```python
from build123d import *

# Parameters (mm, degrees)
SKETCH1_R           = 19.05
BOSS_EXTRUDE1_DEPTH = 34.29
SKETCH3_R           = 10.16
BOSS_EXTRUDE3_DEPTH = 5.08
BOSS_EXTRUDE4_DEPTH = 12.7
FILLET1_R           = 2.54
CHAMFER1_SIZE       = 0.635
SKETCH5_R           = 0.99695
CUT_EXTRUDE1_DEPTH  = 12.7
CHAMFER2_SIZE       = 0.635
CUT_EXTRUDE2_START  = -1.27
SKETCH6_R           = 8.296715315
SKETCH6_R_2         = 3.175
CUT_EXTRUDE2_DEPTH  = 1.27


with BuildPart() as part:
    # Sketch1 → Boss-Extrude1 (new body)
    with BuildSketch(Plane(origin=(0, 0, 0), x_dir=(1, 0, 0), z_dir=(0, 1, 0))):
        with Locations(Location((0, 0, 0), (0, 0, 270))):
            Circle(SKETCH1_R)
    extrude(amount=BOSS_EXTRUDE1_DEPTH)

    # Sketch3 → Boss-Extrude3 (add)
    with BuildSketch(Plane(origin=(0, 34.29, 0), x_dir=(1, 0, 0), z_dir=(0, 1, 0))):
        with Locations(Location((0, 0, 0), (0, 0, 270))):
            Circle(SKETCH3_R)
    extrude(amount=BOSS_EXTRUDE3_DEPTH)

    # Sketch4 → Boss-Extrude4 (add)
    with BuildSketch(Plane(origin=(0, 39.37, 0), x_dir=(1, 0, 0), z_dir=(0, 1, 0))):
        with BuildLine():
            Line((-3.01459652, 0.996409965), (-1.800640593, -2.615017869))
            ThreePointArc((-1.800640593, -2.615017869), (3.009523196, 1.01162994), (-3.01459652, 0.996409965))
        make_face()
    extrude(amount=BOSS_EXTRUDE4_DEPTH)

    # Fillet1
    fillet1_edges = [part.edges().sort_by_distance(p)[0] for p in [
        (0, 0, -19.05),
    ]]
    fillet(fillet1_edges, radius=FILLET1_R)

    # Chamfer1
    chamfer1_edges = [part.edges().sort_by_distance(p)[0] for p in [
        (3.009523196, 52.07, -1.01162994),
    ]]
    chamfer(chamfer1_edges, length=CHAMFER1_SIZE - 0.0001)  # a hair under: the kernel refuses the full size

    # Sketch5 → Cut-Extrude1 (cut)
    with BuildSketch(Plane(origin=(0, 34.29, 0), x_dir=(1, 0, 0), z_dir=(0, 1, 0))):
        with Locations(Location((-11.178825066, -10.636456195, 0), (0, 0, 270))):
            Circle(SKETCH5_R)
        with Locations(Location((-14.999374589, -3.622028738, 0), (0, 0, 270))):
            Circle(SKETCH5_R)
        with Locations(Location((-3.622028738, 14.999374589, 0), (0, 0, 270))):
            Circle(SKETCH5_R)
        with Locations(Location((4.362918394, 14.800853804, 0), (0, 0, 270))):
            Circle(SKETCH5_R)
        with Locations(Location((14.800853804, -4.362918394, 0), (0, 0, 270))):
            Circle(SKETCH5_R)
        with Locations(Location((10.636456195, -11.178825066, 0), (0, 0, 270))):
            Circle(SKETCH5_R)
    extrude(amount=-CUT_EXTRUDE1_DEPTH, mode=Mode.SUBTRACT)

    # Chamfer2
    chamfer2_edges = [part.edges().sort_by_distance(p)[0] for p in [
        (10.636456195, 34.29, 10.181875066),
        (14.800853804, 34.29, 3.365968394),
        (4.362918394, 34.29, -15.797803804),
        (-3.622028738, 34.29, -15.996324589),
        (-14.999374589, 34.29, 2.625078738),
        (-11.178825066, 34.29, 9.639506195),
    ]]
    chamfer(chamfer2_edges, length=CHAMFER2_SIZE)

    # Sketch6 → Cut-Extrude2 (cut)
    with BuildSketch(Plane(origin=(0, 39.37, 0), x_dir=(1, 0, 0), z_dir=(0, 1, 0)).offset(CUT_EXTRUDE2_START)):
        with Locations(Location((0, 0, 0), (0, 0, 270))):
            Circle(SKETCH6_R)
        with Locations(Location((0, 0, 0), (0, 0, 161.709808999))):
            Circle(SKETCH6_R_2, mode=Mode.SUBTRACT)
    extrude(amount=CUT_EXTRUDE2_DEPTH, mode=Mode.SUBTRACT)


solid = part.part
```
Check sheet for the modelled part. Datum: model origin and axes. Units: mm. A direction names the side the tool comes from. Give positions to 0.01 mm unless a question says otherwise; leave off trailing zeros. Write each loop counter-clockwise with the first axis right and the second up, starting at its lowest first coordinate (ties: lowest second). Pieces come first, ordered by that corner, then holes.
Item 1: Cross-section at D-D (y = 45.5). Enter the section's corners in (x, z) (3 decimals), and give its area (3 significant figures).
Item 2: Gauge pin test, flat ends, axial feed: pin 1 (1 mm diameter, centred on x = 10.5, z = 11, fed in from +Y); pin 2 (4 mm diameter, centred on x = 9.5, y = 18.5, fed in from -Z); pin 3 (12 mm diameter, centred on x = 12.5, z = 2, fed in from +Y). Record the tip position at first contact, or that the pin passes through.
Item 3: Cross-section at B-B (y = 32). Enter the section's corners in (x, z), and give its area (3 significant figures).
Item 4: Access from +Z, -Z, +X, -X, +Y, -Y to the whole of each face (thin tool, end or side, straight path). Record for faces 4 (the face through (10.68, 27.707, 10.183)), 5 (the face through (-2.6, 39.37, 0.9)).
Item 5: Cross-section at C-C (z = 0). Enter the section's corners in (x, y) (3 decimals).
Item 6: Cross-section at A-A (x = 0). Enter the section's corners in (y, z) (3 decimals), and give its area (3 significant figures).
Item 7: Draft check along X on faces 1 (the face through (13.828, 27.707, 4.147)), 2 (the face through (-2.416, 45.631, 0.784)), 3 (the face through (-11.59, 18.19, -15.12)). Enter one of: released by +X, released by -X, zero draft, split by the parting line, or undercut.
Item 8: Scan lines: L1, parallel to Y at x = -10, z = -1; L2, parallel to X at y = 32.5, z = 11.5; L3, parallel to Z at x = 10, y = 32.5. Record each from-to range of solid material in increasing order.
Report:
1. outline: (-3.015, -0.996) arc R3.175 ccw (long way) to (-1.801, 2.615) - close
1. area: 30.0 mm2
2. pin 1: stops at y = 21.59
2. pin 2: stops at z = -17.51
2. pin 3: stops at y = 39.37
3. outline: circle Ø38.1 at (0, 0); hole circle Ø1.99 at (-15, 3.62); hole circle Ø1.99 at (-11.18, 10.64); hole circle Ø1.99 at (-3.62, -15); hole circle Ø1.99 at (4.36, -14.8); hole circle Ø1.99 at (10.64, 11.18); hole circle Ø1.99 at (14.8, 4.36)
3. area: 1,120 mm2
4. face 4: +Y
4. face 5: +Z, -X, +Y
5. outline: (-19.05, 2.54) arc R2.54 ccw to (-16.51, 0) - (16.51, 0) arc R2.54 ccw to (19.05, 2.54) - (19.05, 34.29) - (10.16, 34.29) - (10.16, 39.37) - (8.297, 39.37) - (8.297, 38.1) - (3.175, 38.1) - (3.175, 51.435) - (2.54, 52.07) - (-2.54, 52.07) - (-2.68, 51.93) - (-2.68, 39.37) - (-3.175, 39.37) - (-3.175, 38.1) - (-8.297, 38.1) - (-8.297, 39.37) - (-10.16, 39.37) - (-10.16, 34.29) - (-19.05, 34.29) - close
6. outline: (0, -16.51) arc R2.54 ccw to (2.54, -19.05) - (34.29, -19.05) - (34.29, -10.16) - (39.37, -10.16) - (39.37, -8.297) - (38.1, -8.297) - (38.1, -3.175) - (51.435, -3.175) - (52.07, -2.54) - (52.07, 2.54) - (51.435, 3.175) - (38.1, 3.175) - (38.1, 8.297) - (39.37, 8.297) - (39.37, 10.16) - (34.29, 10.16) - (34.29, 19.05) - (2.54, 19.05) arc R2.54 ccw to (0, 16.51) - close
6. area: 1,470 mm2
7. face 1: undercut
7. face 2: released by -X
7. face 3: split by the parting line
8. L1: y = 0 to 39.37
8. L2: x = -15.19 to -11.68, -10.68 to 9.69, 11.58 to 15.19
8. L3: z = -16.21 to 10.41, 11.95 to 16.21
